```python
from build123d import *

# Parameters (mm, degrees)
ESQUISSE1_W                  = 17
ESQUISSE1_H                  = 18
BOSS_EXTRU_1_DEPTH           = 2
ESQUISSE2_W                  = 17
ESQUISSE2_H                  = 18
ESQUISSE2_W_2                = 14
ESQUISSE2_H_2                = 15
BOSS_EXTRU_2_DEPTH           = 5
ESQUISSE3_W                  = 7
ESQUISSE3_H                  = 5
BOSS_EXTRU_3_DEPTH           = 6
ESQUISSE4_R                  = 1.6
ENL_V_MAT_EXTRU_1_DEPTH      = 19.445866746
CHANFREIN1_SIZE              = 1
CHANFREIN1_OF_SYM_TRIE2_SIZE = 1
CHANFREIN2_SIZE              = 1.5
CHANFREIN3_SIZE              = 0.5
ESQUISSE5_R                  = 2.65
ENL_V_MAT_EXTRU_2_DEPTH      = 2
ENL_V_MAT_EXTRU_2_DRAFT      = -3
CHANFREIN4_SIZE              = 0.3
CHANFREIN4_SIZE2             = 0.317026351
CHANFREIN5_SIZE              = 0.5
ESQUISSE6_W                  = 25.293651759
ESQUISSE6_H                  = 13.130697886
ENL_V_MAT_EXTRU_3_DEPTH      = 2


with BuildPart() as part:
    # Esquisse1 → Boss.-Extru.1 (new body)
    with BuildSketch(Plane.XY):
        Rectangle(ESQUISSE1_W, ESQUISSE1_H)
    extrude(amount=BOSS_EXTRU_1_DEPTH)

    # Esquisse2 → Boss.-Extru.2 (add)
    with BuildSketch(Plane.XY.offset(2)):
        Rectangle(ESQUISSE2_W, ESQUISSE2_H)
        Rectangle(ESQUISSE2_W_2, ESQUISSE2_H_2, mode=Mode.SUBTRACT)
    extrude(amount=BOSS_EXTRU_2_DEPTH)

    # Esquisse3 → Boss.-Extru.3 (add)
    with BuildSketch(Plane.ZY.offset(8.5)):
        with Locations((3.5, -2.5)):
            Rectangle(ESQUISSE3_W, ESQUISSE3_H)
    boss_extru_3 = extrude(amount=BOSS_EXTRU_3_DEPTH)

    # Esquisse4 → Enlèv. mat.-Extru.1 (cut, through all)
    with BuildSketch(Plane(origin=(0, 0, 0), x_dir=(1, 0, 0), z_dir=(0, 1, 0))):
        with Locations(Location((-11.8, -3.5, 0), (0, 0, 270))):
            Circle(ESQUISSE4_R)
    enl_v_mat_extru_1 = extrude(amount=-ENL_V_MAT_EXTRU_1_DEPTH, mode=Mode.SUBTRACT)

    # Chanfrein1
    chanfrein1_edges = [part.edges().sort_by_distance(p)[0] for p in [
        (-14.5, -2.5, 0),
        (-14.5, -2.5, 7),
    ]]
    chamfer(chanfrein1_edges, length=CHANFREIN1_SIZE)

    # Symétrie2: Boss.-Extru.3, Enlèv. mat.-Extru.1 across plane
    add(boss_extru_3.mirror(Plane(origin=(0, 0, 0), x_dir=(0, 0, 1), z_dir=(1, 0, 0))))
    add(enl_v_mat_extru_1.mirror(Plane(origin=(0, 0, 0), x_dir=(0, 0, 1), z_dir=(1, 0, 0))), mode=Mode.SUBTRACT)

    # Chanfrein1 of Symétrie2
    chanfrein1_of_sym_trie2_edges = [part.edges().sort_by_distance(p)[0] for p in [
        (14.5, -2.5, 0),
        (14.5, -2.5, 7),
    ]]
    chamfer(chanfrein1_of_sym_trie2_edges, length=CHANFREIN1_OF_SYM_TRIE2_SIZE)

    # Chanfrein2
    chanfrein2_edges = [part.edges().sort_by_distance(p)[0] for p in [
        (-8.5, 9, 3.5),
        (8.5, 9, 3.5),
        (8.5, -9, 3.5),
        (-8.5, -9, 3.5),
    ]]
    chamfer(chanfrein2_edges, length=CHANFREIN2_SIZE)

    # Chanfrein3
    chanfrein3_edges = [part.edges().sort_by_distance(p)[0] for p in [
        (-7, -7.5, 4.5),
        (7, -7.5, 4.5),
        (7, 7.5, 4.5),
        (-7, 7.5, 4.5),
    ]]
    chamfer(chanfrein3_edges, length=CHANFREIN3_SIZE)


with BuildPart() as enl_v_mat_extru_2_tool:
    # Esquisse5 → Enlèv. mat.-Extru.2 (with draft: the straight prism first)
    with BuildSketch(Plane.XY.offset(2)):
        Circle(ESQUISSE5_R)
    extrude(amount=-ENL_V_MAT_EXTRU_2_DEPTH)
    # Enlèv. mat.-Extru.2: the draft: its side faces are tilted about the plane it starts from
    enl_v_mat_extru_2_sides = [enl_v_mat_extru_2_tool.faces().sort_by_distance(p)[0] for p in [
        (-2.65, 0, 1),
    ]]
    draft(enl_v_mat_extru_2_sides, Plane.XY.offset(2), ENL_V_MAT_EXTRU_2_DRAFT)


with BuildPart() as part_1:
    add(part.part)

    # Enlèv. mat.-Extru.2: cut by enl_v_mat_extru_2_tool
    add(enl_v_mat_extru_2_tool.part, mode=Mode.SUBTRACT)

    # Chanfrein4
    chanfrein4_edges = [part_1.edges().sort_by_distance(p)[0] for p in [
        (-2.65, 0, 2),
    ]]
    chanfrein4_side = [part_1.faces().sort_by_distance(p)[0] for p in [
        (0, -7.294817155, 2),
    ]]
    chamfer(chanfrein4_edges, length=CHANFREIN4_SIZE, length2=CHANFREIN4_SIZE2, reference=chanfrein4_side[0])

    # Chanfrein5
    chanfrein5_edges = [part_1.edges().sort_by_distance(p)[0] for p in [
        (-11.8, 0, 1.9),
        (11.8, 0, 1.9),
    ]]
    chamfer(chanfrein5_edges, length=CHANFREIN5_SIZE)

    # Esquisse6 → Enlèv. mat.-Extru.3 (cut)
    with BuildSketch(Plane(origin=(0, 9, 0), x_dir=(1, 0, 0), z_dir=(0, 1, 0))):
        with Locations((1.808818071, -4.181872969)):
            Rectangle(ESQUISSE6_W, ESQUISSE6_H)
    extrude(amount=-ENL_V_MAT_EXTRU_3_DEPTH, mode=Mode.SUBTRACT)


solid = part_1.part
```
Can you work these out from the model? Positions are in its coordinate system, mm. A direction names the side the tool comes from. Round coordinates to 2 decimals unless told otherwise and drop trailing zeros. Loops run counter-clockwise (first coordinate to the right, second up) from the corner with the lowest first, then second, coordinate; pieces in that order, holes last. Notation, with made-up numbers: (-21, -16) -> (35, -16) arc R25 cw to (35, 3) -> close; hole circle Ø5 at (-5.75, -37.75). An arc over 180 degrees is marked (long way). Answer in a Markdown table with one row per item.
Item 1: Suppose I cut it at D-D, the plane y = 5.5. List the corners of the cut face in (x, z) for me, plus the area to 3 significant figures.
Answer block:
| item | result |
|---|---|
| outline | (-8.5, 0) -> (8.5, 0) -> (8.5, 7) -> (7, 7) -> (7, 2) -> (-7, 2) -> (-7, 7) -> (-8.5, 7) -> close |
| area | 49.0 mm² |
Item 2: Suppose I cut it at B-B, the plane x = 11.8. List the corners of the cut face in (y, z) for me.
Answer block:
| item | result |
|---|---|
| outline | (-5, 0) -> (0, 0) -> (0, 1.4) -> (-0.5, 1.9) -> (-5, 1.9) -> close; (-5, 5.1) -> (-0.5, 5.1) -> (0, 5.6) -> (0, 7) -> (-5, 7) -> close |
Item 3: Suppose I cut it at C-C, the plane y = -4.5. List the corners of the cut face in (x, z) for me.
Answer block:
| item | result |
|---|---|
| outline | (-14.5, 1) -> (-13.5, 0) -> (13.5, 0) -> (14.5, 1) -> (14.5, 6) -> (13.5, 7) -> (7, 7) -> (7, 2) -> (-7, 2) -> (-7, 7) -> (-13.5, 7) -> (-14.5, 6) -> close; hole circle Ø3.2 at (-11.8, 3.5); hole circle Ø3.2 at (11.8, 3.5) |
Item 4: If I drill on probe 1 along X at (y, z) = (-1.95, 3.5); probe 2 along Z at (x, y) = (11.8, -2.7); probe 3 along Y at (x, z) = (13.75, 5.5), over which ranges is the centre line in solid material (lowest first)?
Answer block:
| item | result |
|---|---|
| probe 1 | -14.5 to -13.4, -10.2 to -7, 7 to 10.2, 13.4 to 14.5 |
| probe 2 | 0 to 1.9, 5.1 to 7 |
| probe 3 | -5 to 0 |
Item 5: On a 3-axis mill with a long thin cutter (end or side, diameter ignored), from which of +Z, -Z, +X, -X, +Y, -Y can I reach the whole of each face in a straight line? I mean faces 1 (the flat face through (-10, -5, 3)), 2 (the flat face through (7, 0, 4)), 3 (the flat face through (8.5, 3, 3)). Say none if no direction works.
Answer block:
| item | result |
|---|---|
| face 1 | +Z, -Z, -X, -Y |
| face 2 | +Z, +Y |
| face 3 | +Z, -Z, +X, +Y |
Item 6: Will these pins go through, and if not, where does the flat tip stop? P1, Ø3.5, axis at y = 2.5, z = 5, coming from the -X side; P2, Ø4, axis at x = -0.5, y = -3.5, coming from the +Z side; P3, Ø1, axis at y = -7, z = 6, coming from the +X side.
Answer block:
| item | result |
|---|---|
| P1 | x = -8.5 |
| P2 | z = 2 |
| P3 | x = 8.5 |
Item 7: Suppose I cut it at A-A, the plane z = 3.5. Give the number of separate pieces and of enclosed holes in the cut face, plus the area to 3 significant figures.
Answer block:
| item | result |
|---|---|
| separate pieces | 3 |
| enclosed holes | 0 |
| area | 94.5 mm² |
Item 8: We'd pull the mould along Z, two halves only. Please class faces 4 (the flat face through (-14.5, -2, 3)), 5 (the conical face through (-0.56, -2.52, 0.67)), 6 (the cylindrical face through (-13.36, -2.72, 3.15)): released by +Z, released by -Z, zero draft, split by the parting line, or undercut.
Answer block:
| item | result |
|---|---|
| face 4 | zero draft |
| face 5 | released by +Z |
| face 6 | undercut |
